from build123d import *

# Parameters (mm, degrees)
BOSS_EXTRUDE1_DEPTH = 8
SKETCH1_3_R         = 15
SKETCH1_3_R_2       = 6
BOSS_EXTRUDE2_DEPTH = 13
SKETCH2_W           = 72
SKETCH2_H           = 10
BOSS_EXTRUDE3_DEPTH = 22
SKETCH3_R           = 5.1
CUT_EXTRUDE1_DEPTH  = 22
SKETCH4_W           = 72
SKETCH4_H           = 4
BOSS_EXTRUDE4_DEPTH = 5
BOSS_EXTRUDE5_DEPTH = 2.5


with BuildPart() as part:
    # Sketch1 → Boss-Extrude1 (new body)
    with BuildSketch(Plane.XY):
        with BuildLine():
            Line((-36, 10), (-36, 0))
            Line((-36, 0), (36, 0))
            Line((36, 0), (36, 10))
            Line((36, 10), (30, 10))
            ThreePointArc((30, 10), (19.393398282, 14.393398282), (15, 25))
            Line((15, 25), (15, 60))
            ThreePointArc((15, 60), (0, 45), (-15, 60))
            Line((-15, 60), (-15, 25))
            ThreePointArc((-15, 25), (-19.393398282, 14.393398282), (-30, 10))
            Line((-30, 10), (-36, 10))
        make_face()
    extrude(amount=BOSS_EXTRUDE1_DEPTH)

    # Sketch1_3 → Boss-Extrude2 (add)
    with BuildSketch(Plane.XY):
        with Locations((0, 60)):
            Circle(SKETCH1_3_R)
        with Locations(Location((0, 60, 0), (0, 0, 180))):
            Circle(SKETCH1_3_R_2, mode=Mode.SUBTRACT)
    extrude(amount=BOSS_EXTRUDE2_DEPTH)

    # Sketch2 → Boss-Extrude3 (add)
    with BuildSketch(Plane(origin=(0, 0, 0), x_dir=(-1, 0, 0), z_dir=(0, 0, -1))):
        with Locations((0, 5)):
            Rectangle(SKETCH2_W, SKETCH2_H)
    extrude(amount=BOSS_EXTRUDE3_DEPTH)

    # Sketch3 → Cut-Extrude1 (cut)
    with BuildSketch(Plane(origin=(0, 10, 0), x_dir=(1, 0, 0), z_dir=(0, 1, 0))):
        with BuildLine():
            Line((36, 22), (24, 22))
            ThreePointArc((24, 22), (32.485281374, 18.485281374), (36, 10))
            Line((36, 10), (36, 22))
        make_face()
        with Locations(Location((24, 10, 0), (0, 0, 270))):
            Circle(SKETCH3_R)
        with Locations(Location((-24, 10, 0), (0, 0, 270))):
            Circle(SKETCH3_R)
        with BuildLine():
            ThreePointArc((-36, 10), (-32.485281374, 18.485281374), (-24, 22))
            Line((-24, 22), (-36, 22))
            Line((-36, 22), (-36, 10))
        make_face()
    extrude(amount=-CUT_EXTRUDE1_DEPTH, mode=Mode.SUBTRACT)

    # Sketch4 → Boss-Extrude4 (add)
    with BuildSketch(Plane.XY.offset(8)):
        with Locations((0, 2)):
            Rectangle(SKETCH4_W, SKETCH4_H)
    extrude(amount=BOSS_EXTRUDE4_DEPTH)

    # Sketch5 → Boss-Extrude5 (add, symmetric)
    with BuildSketch(Plane(origin=(0, 0, 0), x_dir=(0, 0, -1), z_dir=(1, 0, 0))):
        Polygon((0, 10), (0, 50), (22, 10), align=None)
    extrude(amount=BOSS_EXTRUDE5_DEPTH, both=True)


solid = part.part
CAD build for the part. Positions are in the model's coordinates, mm. A direction names the side the tool comes from. Coordinates: 2 decimals unless noted, no trailing zeros. Loops run counter-clockwise (first coordinate to the right, second up) from the corner with the lowest first, then second, coordinate; pieces in that order, holes last. Notation, with made-up numbers: (-24, -34.75) - (25, -34.75) arc R17 ccw to (25, -26.75) - close; hole circle Ø10 at (86.25, 18.25). An arc over 180 degrees is marked (long way). Write item = value, one per line. Start each with the question number.
Q1. Flat gauge pins, fed straight in: pin 1 Ø2.5 at (y, z) = (49.5, 6) entering from -X; pin 2 Ø2.5 at (y, z) = (46.5, 4.5) entering from +X; pin 3 Ø1 at (x, z) = (-23.5, -16) entering from -Y; pin 4 Ø12 at (x, z) = (-18, -7.5) entering from +Y. Where does each tip first touch, or does it go through?
Q2. Cut at B-B, the plane z = 1. List the corners of the cut face in (x, y).
Q3. Cut at D-D, the plane z = -11. List the corners of the cut face in (x, y).
Q4. Pull direction Y, two halves, no side cores. Call faces 4 (the cylindrical face through (19.51, 14.28, 3.94)), 5 (the flat face through (15, 42, 4)), 6 (the cylindrical face through (1.301, 65.857, 6.409)): pulls with the +Y half, pulls with the -Y half, needs draft (parallel to the pull), parting line crosses it, or undercut.
Q5. Cut at C-C, the plane z = 11. List the corners of the cut face in (x, y).
Q6. Drill centre lines: L1, parallel to Y at x = 0, z = 9; L2, parallel to X at y = 4, z = -10; L3, parallel to Y at x = 0, z = 5. Where is each one in solid material? Low to high.
Q7. Cut at A-A, the plane x = 0. List the corners of the cut face in (y, z).
Q8. Which spindle directions (+Z, -Z, +X, -X, +Y, -Y) get a long thin tool onto all of the face, cutting with end or side? Do faces 1 (the flat face through (-2.5, 21, -6)), 2 (the cylindrical face through (-1.953, 74.872, 7.853)), 3 (the flat face through (19, 10, -7)). Say none if no direction does.
Computed:
q1.pin_1 = -15
q1.pin_2 = 15
q1.pin_3 = 0
q1.pin_4 = 10
q2.outline = (-36, 0) - (36, 0) - (36, 10) - (30, 10) arc R15 cw to (15, 25) - (15, 60) arc R15 ccw to (-15, 60) - (-15, 25) arc R15 cw to (-30, 10) - (-36, 10) - close; hole circle Ø12 at (0, 60)
q3.outline = (-35.96, 0) - (-29, 0) - (-29, 10) - (-35.96, 10) - close; (-19, 0) - (19, 0) - (19, 10) - (2.5, 10) - (2.5, 30) - (-2.5, 30) - (-2.5, 10) - (-19, 10) - close; (29, 0) - (35.96, 0) - (35.96, 10) - (29, 10) - close
q4.face_4 = pulls with the +Y half
q4.face_5 = needs draft
q4.face_6 = undercut
q5.outline = (-36, 0) - (36, 0) - (36, 4) - (-36, 4) - close; circle Ø30 at (0, 60); hole circle Ø12 at (0, 60)
q6.L1 = 0 to 4, 45 to 54, 66 to 75
q6.L2 = -36 to -29.1, -18.9 to 18.9, 29.1 to 36
q6.L3 = 0 to 54, 66 to 75
q7.outline = (0, -22) - (10, -22) - (50, 0) - (54, 0) - (54, 13) - (45, 13) - (45, 8) - (4, 8) - (4, 13) - (0, 13) - close; (66, 0) - (75, 0) - (75, 13) - (66, 13) - close
q8.face_1 = -Z, -X, +Y
q8.face_2 = +Z
q8.face_3 = -Z, +X, +Y
